Autodesk Inventor part; units mm, degrees
ref_plane "YZ Plane" through (0, 0, 0) normal (1, 0, 0) x (0, 1, 0)
ref_plane "XZ Plane" through (0, 0, 0) normal (0, 1, 0) x (-1, 0, 0)
ref_plane "XY Plane" through (0, 0, 0) normal (0, 0, 1) x (1, 0, 0)
sketch "Sketch1" plane through (0, 0, 0) normal (0, 1, 0) x (-1, 0, 0)
  line L0 (0, 0) -> (37.592, 0)
  line L1 (37.592, 0) -> (37.592, 37.465)
  line L2 (37.592, 37.465) -> (0, 37.465)
  line L3 (0, 37.465) -> (0, 0)
  line L4 (37.592, 18.7325) -> (26.289, 18.7325)
  line L5 (37.592, 18.7325) -> (48.895, 18.7325) construction
  circle A0 centre (26.289, 18.7325) radius 2.3241
  circle A1 centre (14.224, 18.7325) radius 2.3241
  line L6 (34.6202, 34.4932) -> (34.6202, 2.9718)
  line L7 (34.6202, 2.9718) -> (2.9718, 2.9718)
  line L8 (2.9718, 2.9718) -> (2.9718, 34.4932)
  line L9 (2.9718, 34.4932) -> (34.6202, 34.4932)
  dimension "d0" = 37.592
  dimension "d1" = 37.465
  dimension "d2" = 11.303
  dimension "d3" = 180
  dimension "d4" = 4.6482
  dimension "d7" = 12.065
  dimension "d14" = 2.9718
extrude "Extrusion1" add sketch "Sketch1" along normal blind 3.175 contours L6 L7 L8 L9 | L3 L2 L1 L0
extrude "Extrusion2" cut sketch "Sketch1" along normal blind 1.5875 contours L6 L7 L8 L9
properties part number "gps sensor holder"
Can you work these out from the model? Positions are in its coordinate system, mm. A direction names the side the tool comes from. Round coordinates to 2 decimals unless told otherwise and drop trailing zeros. Write each loop counter-clockwise with the first axis right and the second up, starting at its lowest first coordinate (ties: lowest second). Pieces come first, ordered by that corner, then holes. Notation, with made-up numbers: (-26, -2.75) -> (32, -2.75) arc R14 ccw to (32, 20.25) -> close; hole circle Ø1 at (26, 64). An arc over 180 degrees is marked (long way). One line per question, with ' | ' between items. Start each with the question number.
1) Suppose I cut it at B-B on x = -13. Write out the boundary of the cut face in (y, z) (1 decimal).
2) If we mould it in two halves opening along Z, with no side actions, what happens to faces 3 (the flat face through (-19, 1.588, 19)), 4 (the flat face through (-19, 2, 0)), 5 (the flat face through (-19, 0, 2)), 6 (the flat face through (-34.62, 1, 19))? For each: released by +Z, released by -Z, zero draft, split by the parting line, or undercut.
3) I need wall thicknesses on line 1 (Z direction, x = -8, y = 1.45) (3 decimals); line 2 (X direction, y = 2.8, z = 20); line 3 (X direction, y = 0.5, z = 26.5). Which ranges of each line are inside material? Lowest first, please. Write a range as [from, to].
4) On a 3-axis mill with a long thin cutter (end or side, diameter ignored), from which of +Z, -Z, +X, -X, +Y, -Y can I reach the whole of each face in a straight line? I mean faces 1 (the cylindrical face through (-16.44, 2.37, 18.03)), 2 (the flat face through (-19, 1, 34.493)). Say none if no direction works.
5) I'm going to push flat-ended pins straight in: P1, Ø1, axis at x = -30.5, z = 8.5, coming from the -Y side; P2, Ø0.5, axis at y = 0.5, z = 24, coming from the +X side. Where does each tip first touch, or does it pass through?
6) Suppose I cut it at A-A on y = 1. Write out the boundary of the cut face in (x, z) (3 decimals), then the cut area to 3 significant figures.
7) Suppose I cut it at D-D on x = -26. Write out the boundary of the cut face in (y, z) (1 decimal), then the cut area to 3 significant figures.
8) Suppose I cut it at C-C on z = 27.5. Write out the boundary of the cut face in (x, y) (1 decimal), then the cut area to 3 significant figures.
Return value:
1) outline: (0, 0) -> (3.2, 0) -> (3.2, 16.8) -> (1.6, 16.8) -> (1.6, 3) -> (0, 3) -> close; (0, 34.5) -> (1.6, 34.5) -> (1.6, 20.7) -> (3.2, 20.7) -> (3.2, 37.5) -> (0, 37.5) -> close
2) face 3: undercut | face 4: released by -Z | face 5: zero draft | face 6: undercut
3) line 1: z = [0, 2.972], [34.493, 37.465] | line 2: x = [-37.59, -28.24], [-24.34, -16.17], [-12.28, 0] | line 3: x = [-37.59, -34.62], [-2.97, 0]
4) face 1: +Y, -Y | face 2: -Y
5) P1: stops at y = 1.59 | P2: stops at x = 0
6) outline: (-37.592, 0) -> (0, 0) -> (0, 37.465) -> (-37.592, 37.465) -> close; hole (-34.62, 2.972) -> (-2.972, 2.972) -> (-2.972, 34.493) -> (-34.62, 34.493) -> close | area: 411 mm2
7) outline: (0, 0) -> (3.2, 0) -> (3.2, 16.4) -> (1.6, 16.4) -> (1.6, 3) -> (0, 3) -> close; (0, 34.5) -> (1.6, 34.5) -> (1.6, 21) -> (3.2, 21) -> (3.2, 37.5) -> (0, 37.5) -> close | area: 61.6 mm2
8) outline: (-37.6, 0) -> (-34.6, 0) -> (-34.6, 1.6) -> (-3, 1.6) -> (-3, 0) -> (0, 0) -> (0, 3.2) -> (-37.6, 3.2) -> close | area: 69.1 mm2
